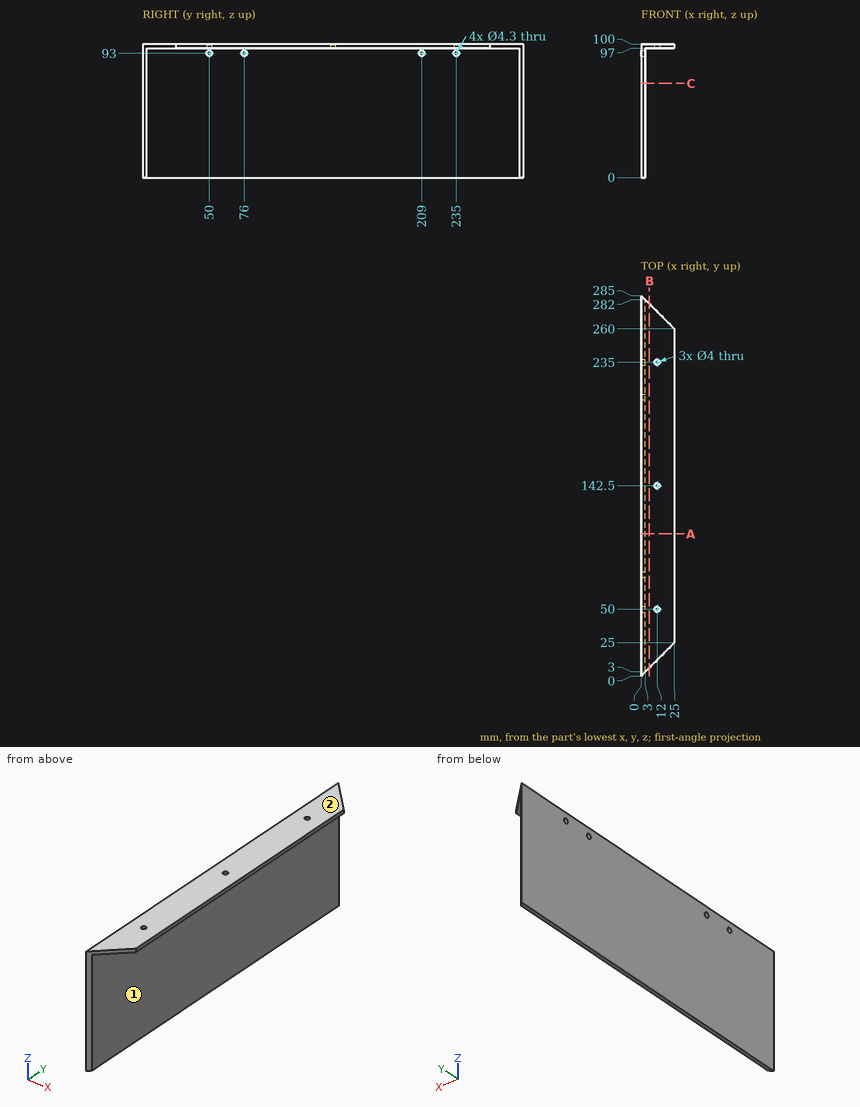
Could you check a few things on this drawing? It's one solid part, dimensions in mm from its lowest x, y, z. A direction names the side the tool comes from. Coordinates: 2 decimals unless noted, no trailing zeros. Order: outer loops, then holes, each group sorted by start corner. A loop starts at its lowest first (then second) coordinate and runs counter-clockwise, first axis right, second up.
1. If we section it at A-A (y = 106.5): Please give me the cut outline in (x, z).
2. I'm going to push flat-ended pins straight in: pin 1 (12 mm diameter, centred on x = 6.5, z = 26.5, fed in from -Y); pin 2 (1 mm diameter, centred on y = 155.5, z = 67.5, fed in from +X); pin 3 (11 mm diameter, centred on x = 17.5, y = 191, fed in from -Z). Where does each tip first touch, or does it pass through?
3. If we section it at C-C (z = 70.5): Please give me the cut outline in (x, y).
4. I need wall thicknesses on line 1 (Z direction, x = 1.6, y = 76); line 2 (Y direction, x = 12, z = 99.45); line 3 (Y direction, x = 1, z = 93). Which ranges of each line are inside material? Lowest first, please.
5. If we section it at B-B (x = 6.25): Please give me the cut outline in (y, z), then the cut area to 4 significant figures.
6. For the marked faces 1 and 2, which set-ups out of +Z, -Z, +X, -X, +Y, -Y let a thin tool reach every point of the face, with its end or its side?
Entries:
1. outline: (0, 0) - (3, 0) - (3, 97) - (25, 97) - (25, 100) - (0, 100) - close
2. pin 1: stops at y = 0.5
2. pin 2: stops at x = 3
2. pin 3: stops at z = 97
3. outline: (0, 0) - (3, 3) - (3, 282) - (0, 285) - close
4. line 1: z = 0 to 90.85, 95.15 to 100
4. line 2: y = 12 to 48, 52 to 140.5, 144.5 to 233, 237 to 273
4. line 3: y = 1 to 47.85, 52.15 to 73.85, 78.15 to 206.85, 211.15 to 232.85, 237.15 to 284
5. outline: (6.25, 97) - (278.75, 97) - (278.75, 100) - (6.25, 100) - close
5. area: 817.5 mm2
6. face 1: -Z, +X, +Y, -Y
6. face 2: +Z, +X, -X, +Y, -Y
